Work out the finished part from the listing and answer in its coordinate system (mm). A direction names the side the tool comes from. Round coordinates to 2 decimals unless told otherwise and drop trailing zeros. Order: outer loops, then holes, each group sorted by start corner. A loop starts at its lowest first (then second) coordinate and runs counter-clockwise, first axis right, second up. Notation, with made-up numbers: (30.25, 51) - (82.25, 51) arc R26 ccw to (82.25, 86) - close; hole circle Ø1 at (24, 46). An arc over 180 degrees is marked (long way). One line per question, with ' | ' between items. Start each with the question number.
from build123d import *

# Parameters (mm, degrees)
CUT_EXTRUDE1_DEPTH      = 6
CIRPATTERN1_COUNT       = 16
CUT_EXTRUDE2_REACH      = 15.574
CUT_EXTRUDE2_END_RADIUS = 8
SKETCH3_R               = 1.65
CUT_EXTRUDE3_REACH      = 15.574
CUT_EXTRUDE3_END_RADIUS = 8
SKETCH4_R               = 1.65
SKETCH5_R               = 6.1
SKETCH5_R_2             = 6
CUT_EXTRUDE_THIN1_DEPTH = 5
CHAMFER1_SIZE           = 1


with BuildPart() as part:
    # Skica2 → Revolute (revolve)
    with BuildSketch(Plane.XY):
        Polygon((8, 7.5), (3, 7.5), (3, -7.5), (6.11, -7.5), (6.11, -6.5), (8, -6.5), (8, -5.5), (6.11, -5.5), (6.11, 0.5), (8, 0.5), align=None)
    revolve(axis=Axis((0, -7.5, 0), (0, 1, 0)))

    # Sketch2 → Cut-Extrude1 (cut)
    with BuildSketch(Plane.XZ.offset(-0.5)):
        with BuildLine():
            ThreePointArc((-1.285657138, 5.973205649), (-0.969411866, 5.937681099), (-0.73865565, 5.718535862))
            ThreePointArc((-0.73865565, 5.718535862), (0, 5.27402372), (0.73865565, 5.718535862))
            ThreePointArc((0.73865565, 5.718535862), (0.969411866, 5.937681099), (1.285657138, 5.973205649))
            ThreePointArc((1.285657138, 5.973205649), (0, 6.11), (-1.285657138, 5.973205649))
        make_face()
    cut_extrude1 = extrude(amount=CUT_EXTRUDE1_DEPTH, mode=Mode.SUBTRACT)

    # CirPattern1: Cut-Extrude1 ×16 about axis
    cirpattern1_axis = Axis((0, 0, 0), (0, 1, 0))
    for i in range(1, CIRPATTERN1_COUNT):
        add(cut_extrude1.rotate(cirpattern1_axis, i * 360 / CIRPATTERN1_COUNT), mode=Mode.SUBTRACT)

    # Cut-Extrude2: up to this cylinder (the profile starts inside it)
    cut_extrude2_end = Plane(origin=(0, 4, 0), z_dir=(0, -1, 0)) * Cylinder(CUT_EXTRUDE2_END_RADIUS, 48.148, mode=Mode.PRIVATE)
    # Sketch3 → Cut-Extrude2 (cut, up to the surface)
    with BuildSketch(Plane(origin=(0, 0, 0), x_dir=(0, 0, -1), z_dir=(1, 0, 0)), mode=Mode.PRIVATE) as cut_extrude2_sk1:
        with Locations((0, 4)):
            Circle(SKETCH3_R)
    cut_extrude2_tool1 = extrude(cut_extrude2_sk1.sketch, amount=-CUT_EXTRUDE2_REACH, mode=Mode.PRIVATE) & cut_extrude2_end
    add(cut_extrude2_tool1.solids().sort_by_distance((0, 4, 0))[0], mode=Mode.SUBTRACT)

    # Cut-Extrude3: up to this cylinder (the profile starts inside it)
    cut_extrude3_end = Plane(origin=(0, 4, 0), z_dir=(0, -1, 0)) * Cylinder(CUT_EXTRUDE3_END_RADIUS, 48.148, mode=Mode.PRIVATE)
    # Sketch4 → Cut-Extrude3 (cut, up to the surface)
    with BuildSketch(Plane.XY, mode=Mode.PRIVATE) as cut_extrude3_sk1:
        with Locations((0, 4)):
            Circle(SKETCH4_R)
    cut_extrude3_tool1 = extrude(cut_extrude3_sk1.sketch, amount=-CUT_EXTRUDE3_REACH, mode=Mode.PRIVATE) & cut_extrude3_end
    add(cut_extrude3_tool1.solids().sort_by_distance((0, 4, 0))[0], mode=Mode.SUBTRACT)

    # Sketch5 → Cut-Extrude-Thin1 (cut)
    with BuildSketch(Plane(origin=(0, 7.5, 0), x_dir=(1, 0, 0), z_dir=(0, 1, 0))):
        Circle(SKETCH5_R)
        Circle(SKETCH5_R_2, mode=Mode.SUBTRACT)
    extrude(amount=-CUT_EXTRUDE_THIN1_DEPTH, mode=Mode.SUBTRACT)

    # Chamfer1
    chamfer1_edges = [part.edges().sort_by_distance(p)[0] for p in [
        (-6.11, -6.5, 0),
    ]]
    chamfer(chamfer1_edges, length=CHAMFER1_SIZE - 0.0001)  # a hair under: the kernel refuses the full size


solid = part.part
1) Flat-ended cylindrical pins translate along their axes: pin 1 (1.5 mm diameter, centred on x = -1.5, y = -1.5, fed in from +Z); pin 2 (5.5 mm diameter, centred on x = 0, y = 4, fed in from -Z); pin 3 (2 mm diameter, centred on x = -2.5, y = 4.5, fed in from -Z); pin 4 (1.5 mm diameter, centred on x = 1, y = -5, fed in from +Z). Find the tip coordinate at first contact, or state that the pin passes through.
2) Section A-A on x = 0 is taken. Give the number of separate pieces and of enclosed holes in the cut face, and give its area (3 significant figures).
3) For faces 1 (the cylindrical face through (-4.868, -2.458, -2.03)), 2 (the cylindrical face through (0.013, -2.458, -5.274)), 3 (the cylindrical face through (4.868, -2.458, 2.03)), 4 (the flat face through (5.2, -5.5, -1.9)), 5 (the cylindrical face through (1.384, -0.105, 2.662)), determine the directions among +Z, -Z, +X, -X, +Y, -Y from which every point of the face is accessible in a straight line to the end or side of a thin tool.
4) Straight lines are drawn through the part: line 1 (Y direction, x = -5.75, z = 0); line 2 (X direction, y = 0.75, z = 0); line 3 (Y direction, x = 0, z = -6.7). For each, find the intervals that lie inside material, in ascending order.
5) Determine the mould class of faces 6 (the cylindrical face through (-1.73, -5.99, 7.81)), 7 (the cylindrical face through (3.72, -2.46, 3.74)), 8 (the cylindrical face through (-2.03, -2.458, 4.868)), 9 (the cylindrical face through (-2.007, -2.458, -4.878)) for opening direction Z: released by +Z, released by -Z, zero draft, split by the parting line, or undercut.
6) Section C-C on y = 4 is taken. Give the vertices of the cut face in (x, z), and give its area (3 significant figures).
7) Section D-D on y = 2 is taken. Give the vertices of the cut face in (x, z).
Recorded:
1) pin 1: stops at z = 5.98 | pin 2: stops at z = -8 | pin 3: stops at z = -7.86 | pin 4: stops at z = 7.99
2) separate pieces: 4 | enclosed holes: 0 | area: 97.3 mm²
3) face 1: -X | face 2: -Z | face 3: +X | face 4: none | face 5: +Y, -Y
4) line 1: y = -7.5 to -5.5, 0.5 to 2.35, 5.65 to 7.5 | line 2: x = -8 to -3, 3 to 8 | line 3: y = -6.91 to -5.5, 0.5 to 2.35, 5.65 to 7.5
5) face 6: split by the parting line | face 7: undercut | face 8: released by +Z | face 9: released by -Z
6) outline: (-7.83, -1.65) arc R8 ccw to (-1.65, -7.83) - (-1.65, -5.87) arc R6.1 cw to (-5.87, -1.65) - close; (-7.83, 1.65) - (-5.87, 1.65) arc R6.1 cw (long way) to (1.65, -5.87) - (1.65, -7.83) arc R8 ccw (long way) to start; (-5.77, -1.65) arc R6 ccw to (-1.65, -5.77) - (-1.65, -2.51) arc R3 cw to (-2.51, -1.65) - close; (-5.77, 1.65) - (-2.51, 1.65) arc R3 cw (long way) to (1.65, -2.51) - (1.65, -5.77) arc R6 ccw (long way) to start | area: 136 mm²
7) outline: circle Ø16 at (0, 0); hole circle Ø6 at (0, 0)
